The model under review builds one solid part; all positions refer to its coordinate system, in mm. Face numbers are marked on the shaded views. A direction names the side the tool comes from. Round coordinates to 2 decimals unless told otherwise and drop trailing zeros. Loops run counter-clockwise (first coordinate to the right, second up) from the corner with the lowest first, then second, coordinate; pieces in that order, holes last. Notation, with made-up numbers: M -16.5,88.25 L 14.5,88.25 A22 cw 14.5,99.25 Z; hole C 36.25,60 d8. An arc over 180 degrees is marked long. One line per question, with ' | ' between items.
from build123d import *

# Parameters (mm, degrees)
EXTRUDE_1_DEPTH = 3
SKETCH_2_R      = 2
EXTRUDE_2_DEPTH = 5


with BuildPart() as part:
    # 草图1 → 凸台-拉伸1 (new body)
    with BuildSketch(Plane.XY):
        Polygon((1.537378268, -3.104266107), (3.457062442, -0.220724418), (1.919684175, 2.883541688), (-1.537378268, 3.104266107), (-3.457062442, 0.220724418), (-1.919684175, -2.883541688), align=None)
    extrude(amount=EXTRUDE_1_DEPTH)

    # 草图2 → 凸台-拉伸2 (add)
    with BuildSketch(Plane(origin=(0, 0, 0), x_dir=(-1, 0, 0), z_dir=(0, 0, -1))):
        Circle(SKETCH_2_R)
    extrude(amount=EXTRUDE_2_DEPTH)


solid = part.part
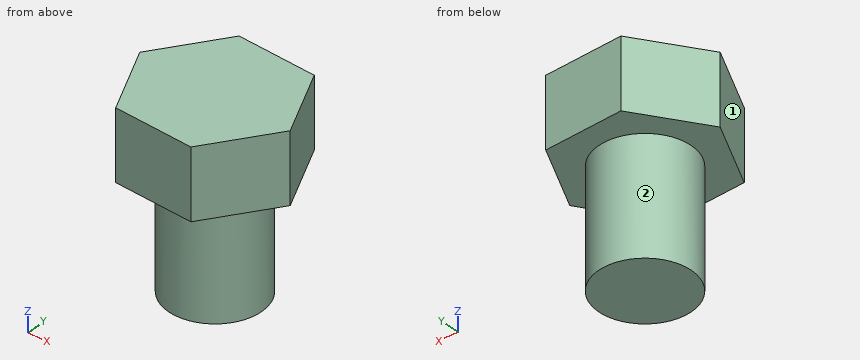
1) Add section A-A on y = 0. State the section outline as (x, z) points.
Output values:
outline: M -3.35,0 L -2,0 L -2,-5 L 2,-5 L 2,0 L 3.35,0 L 3.35,3 L -3.35,3 Z
2) For line 1 (Z direction, x = 2.25, y = -0.5); line 2 (Y direction, x = -2.25, z = 0.75); line 3 (X direction, y = -1, z = -0.5), list the stretches that pass through material, from the lowest coordinate up.
Output values:
line 1: z = 0 to 3 | line 2: y = -2.22 to 2.03 | line 3: x = -1.73 to 1.73
3) Insertion check: P1, Ø1, axis at y = 1.5, z = 0.5, coming from the +X side. The pin has a flat end and moves straight along its axis. Give the tip position at first contact, or say it passes through.
Output values:
P1: stops at x = 2.85
4) Add section C-C on z = -2.75. State the section outline as (x, y) points, then the cut area to 3 significant figures.
Output values:
outline: C 0,0 d4 | area: 12.6 mm²
5) Add section D-D on z = 0.5. State the section outline as (x, y) points.
Output values:
outline: M -3.46,0.22 L -1.92,-2.88 L 1.54,-3.1 L 3.46,-0.22 L 1.92,2.88 L -1.54,3.1 Z
6) Add section B-B on x = 0. State the section outline as (y, z) points, then the cut area to 3 significant figures.
Output values:
outline: M -3.01,0 L -2,0 L -2,-5 L 2,-5 L 2,0 L 3.01,0 L 3.01,3 L -3.01,3 Z | area: 38.0 mm²
7) Machinability: for the marked faces 1 and 2, which of the approach directions +Z, -Z, +X, -X, +Y, -Y give a long, thin tool a straight path to every point of the face, cutting with its end or side? Answer none if there is none.
Output values:
face 1: +Z, -Z, -X, -Y | face 2: -Z
